Geometry: final body of the model. Coordinates: model frame, mm. Face numbers are marked on the shaded views. Coordinates: 2 decimals unless noted, no trailing zeros. Write each loop counter-clockwise with the first axis right and the second up, starting at its lowest first coordinate (ties: lowest second). Pieces come first, ordered by that corner, then holes. Notation, with made-up numbers: (46, 76) -> (53, 76) arc R28 ccw to (53, 95) -> close; hole circle Ø11 at (31, 0). An arc over 180 degrees is marked (long way). One line per item, written item: value.
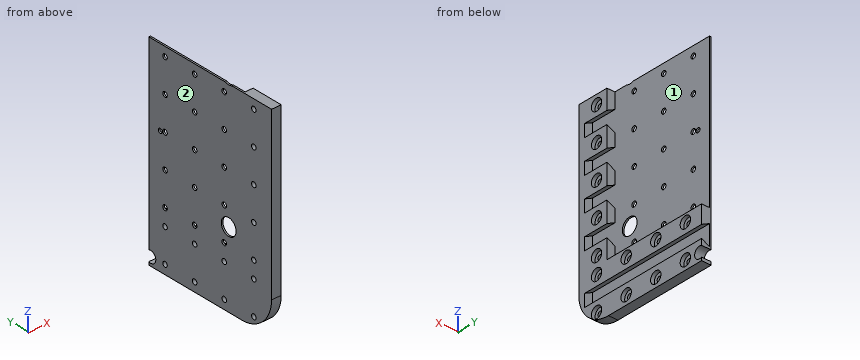
Autodesk Inventor part; units mm, degrees
ref_plane "YZ Plane" through (0, 0, 0) normal (1, 0, 0) x (0, 1, 0)
ref_plane "XZ Plane" through (0, 0, 0) normal (0, 1, 0) x (-1, 0, 0)
ref_plane "XY Plane" through (0, 0, 0) normal (0, 0, 1) x (1, 0, 0)
sketch "Sketch1" plane through (0, 0, 0) normal (0, 1, 0) x (-1, 0, 0)
  line L0 (7.366, 6.1452) -> (7.366, -23.8548)
  line L1 (7.366, -23.8548) -> (0, -23.8548)
  line L2 (6.096, -8.0476) -> (6.096, -9.0212)
  line L3 (0, 0.4868) -> (0, 3.5348)
  line L4 (6.096, 3.5348) -> (6.096, -8.0476)
  line L5 (0, -9.0212) -> (0, -11.8152)
  line L6 (6.096, -12.0692) -> (6.096, -9.0212)
  line L7 (6.096, 3.5348) -> (0, 0.4868)
  line L8 (6.096, -12.0692) -> (0, -9.0212)
  line L9 (0, -23.8548) -> (0, -9.0212)
  line L10 (0, 0.4868) -> (0, 16.3788)
  line L11 (6.096, 13.3308) -> (6.096, 16.3788)
  line L12 (6.096, 13.3308) -> (0, 16.3788)
  line L13 (6.096, 28.9348) -> (6.096, 17.3524)
  line L14 (6.096, 28.9348) -> (0, 25.8868)
  line L15 (6.096, 17.3524) -> (6.096, 16.3788)
  line L16 (6.096, 38.7308) -> (6.096, 41.7788)
  line L17 (6.096, 38.7308) -> (0, 41.7788)
  line L18 (6.096, 54.3348) -> (6.096, 42.7524)
  line L19 (6.096, 54.3348) -> (0, 51.2868)
  line L20 (6.096, 42.7524) -> (6.096, 41.7788)
  line L21 (6.096, 64.1308) -> (6.096, 67.1788)
  line L22 (6.096, 64.1308) -> (0, 67.1788)
  line L23 (6.096, 79.7348) -> (6.096, 68.1524)
  line L24 (6.096, 79.7348) -> (0, 76.6868)
  line L25 (6.096, 68.1524) -> (6.096, 67.1788)
  line L26 (7.366, 6.1452) -> (7.366, 91.622)
  line L27 (7.366, 91.622) -> (0, 91.622)
  line L28 (0, 25.8868) -> (0, 41.7788)
  line L29 (0, 51.2868) -> (0, 67.1788)
  line L30 (0, 76.6868) -> (0, 91.622)
  line L31 (6.096, -4.2672) -> (4.0009, -4.2672) construction
  point P0 (0, 0)
  dimension "d0" = 7.366
  dimension "d8" = 9.508
  dimension "d10" = 3.048
  dimension "d11" = 3.048
  dimension "d12" = 6.096
  dimension "d17" = 25.4
  dimension "d24" = 11.7856
  dimension "d67" = 115.4768
  dimension "d70" = 23.8548
  dimension "d71" = 4.754
extrude "MultipleTeeth" add sketch "Sketch1" along normal blind 19.05
sketch "Sketch2" plane through (0, 0, 0) normal (0, -1, 0) x (1, 0, 0)
  line L0 (0, 0.4868) -> (-6.096, 3.5348) construction
  line L1 (-6.096, 3.5348) -> (-6.096, -12.0692) construction
  line L2 (-6.096, -12.0692) -> (0, -9.0212) construction
  line L3 (0, 16.3788) -> (0, 0.4868)
  line L4 (0, 0.4868) -> (-6.096, 3.5348)
  line L5 (-6.096, -12.0692) -> (0, -9.0212)
  line L6 (-6.096, 3.5348) -> (-6.096, -12.0692)
  line L7 (-6.096, -12.0692) -> (-6.096, 3.5348)
  line L8 (0, -9.0212) -> (-6.096, -12.0692)
  line L9 (-7.366, -23.8548) -> (-7.366, 91.622)
  line L10 (-7.366, -59.508) -> (-7.366, -32.8548)
  line L11 (-7.366, -23.8548) -> (0, -23.8548)
  line L12 (-7.366, 91.622) -> (0, 91.622)
  line L13 (-7.366, -55.8503) -> (-7.366, -40.458) construction
  line L14 (0, -43.0234) -> (0, -59.508) construction
  line L15 (-6.096, -62.0648) -> (0, -62.0648) construction
  line L16 (0, -32.8548) -> (0, -37.6258)
  line L17 (0, -49.9828) -> (0, -62.0648)
  line L18 (0, -62.0648) -> (0, -59.508)
  line L19 (0, -32.8548) -> (-7.366, -32.8548) construction
  line L20 (0, -51.9048) -> (-7.366, -51.9048) construction
  line L21 (0, -42.3798) -> (-7.366, -42.3798) construction
  line L22 (-6.096, -12.0692) -> (-6.096, -62.0648) construction
  line L23 (0, -37.6258) -> (-6.096, -34.5778)
  line L24 (-6.096, -50.1818) -> (-6.096, -34.5778)
  line L25 (0, -47.1338) -> (-6.096, -50.1818)
  line L26 (0, -9.0212) -> (0, -23.8548)
  line L27 (0, -23.8548) -> (0, -32.8548)
  line L28 (-7.366, -32.8548) -> (-7.366, -23.8548)
  line L29 (0, -49.9828) -> (0, -47.1338)
  line L30 (0, -62.0648) -> (-7.366, -62.0648)
  line L31 (-7.366, -62.0648) -> (-7.366, -59.508)
  point P0 (0, 0)
  dimension "d25" = 115.4768
  dimension "d33" = 9
  dimension "d34" = 19.05
  dimension "d36" = 9.525
  dimension "d38" = 10.16
extrude "LongTooth" add sketch "Sketch2" against normal blind 100.2792
sketch "Sketch3" plane through (0, 19.05, 0) normal (0, 1, 0) x (1, 0, 0)
  line L0 (-6.096, -3.5348) -> (-6.096, 12.0692) construction
  line L1 (0, 23.8548) -> (-7.366, 23.8548)
  line L2 (-7.366, -91.622) -> (0, -91.622)
  line L3 (-7.366, 23.8548) -> (-6.096, 23.8548)
  line L4 (-6.096, 23.8548) -> (-6.096, -91.622)
  line L5 (-6.096, -91.622) -> (-7.366, -91.622)
  line L6 (-7.366, -91.622) -> (-7.366, 23.8548)
  point P0 (0, 0)
extrude "ThinPlate" add sketch "Sketch3" along normal up to surface (81.2292 mm away)
sketch "Sketch4" plane through (0, 0, 0) normal (0, -1, 0) x (1, 0, 0)
  line L0 (-6.096, 91.622) -> (0, 91.622)
  line L1 (-7.366, 91.622) -> (-7.366, -62.0648)
  line L2 (0, 91.622) -> (-7.366, 91.622)
  line L3 (-7.366, 91.622) -> (-7.366, -62.0648)
  line L4 (-7.366, -62.0648) -> (0, -62.0648)
  line L5 (0, -62.0648) -> (0, 91.622)
  point P0 (0, 0)
extrude "Extrusion4" add sketch "Sketch4" along normal blind 5.08
ref_plane "Work Plane1" through (-15.892, 0, 8.4328) normal (0, 0, 1) x (0, 1, 0)
sketch "Sketch6" plane through (0, 19.05, 16.3788) normal (1, 0, 0) x (0, 0, -1)
  circle A0 centre (71.4586, -8.89) radius 1.9304
  line L0 (78.4436, -24.13) -> (78.4436, 81.2292)
  line L1 (78.4436, -24.13) -> (-75.2432, -24.13)
  circle A1 centre (58.7586, -8.89) radius 1.9304
  circle A2 centre (46.0586, -8.89) radius 1.9304
  circle A3 centre (71.4586, 3.81) radius 1.9304
  circle A4 centre (58.7586, 3.81) radius 1.9304
  circle A5 centre (46.0586, 3.81) radius 1.9304
  circle A6 centre (71.4586, 16.51) radius 1.9304
  circle A7 centre (58.7586, 16.51) radius 1.9304
  circle A8 centre (46.0586, 16.51) radius 1.9304
  circle A9 centre (71.4586, 29.21) radius 1.9304
  circle A10 centre (58.7586, 29.21) radius 1.9304
  circle A11 centre (46.0586, 29.21) radius 1.9304
  circle A12 centre (71.4586, 41.91) radius 1.9304
  circle A13 centre (58.7586, 41.91) radius 1.9304
  circle A14 centre (46.0586, 41.91) radius 1.9304
  circle A15 centre (71.4586, 54.61) radius 1.9304
  circle A16 centre (58.7586, 54.61) radius 1.9304
  circle A17 centre (46.0586, 54.61) radius 1.9304
  circle A18 centre (71.4586, 67.31) radius 1.9304
  circle A19 centre (58.7586, 67.31) radius 1.9304
  circle A20 centre (46.0586, 67.31) radius 1.9304
  circle A21 centre (33.3586, -8.89) radius 1.9304
  circle A22 centre (33.3586, 3.81) radius 1.9304
  circle A23 centre (33.3586, 16.51) radius 1.9304
  circle A24 centre (33.3586, 29.21) radius 1.9304
  circle A25 centre (33.3586, 41.91) radius 1.9304
  circle A26 centre (33.3586, 54.61) radius 1.9304
  circle A27 centre (33.3586, 67.31) radius 1.9304
  circle A28 centre (20.6586, -8.89) radius 1.9304
  circle A29 centre (20.6586, 3.81) radius 1.9304
  circle A30 centre (20.6586, 16.51) radius 1.9304
  circle A31 centre (20.6586, 29.21) radius 1.9304
  circle A32 centre (20.6586, 41.91) radius 1.9304
  circle A33 centre (20.6586, 54.61) radius 1.9304
  circle A34 centre (20.6586, 67.31) radius 1.9304
  circle A35 centre (7.9586, -8.89) radius 1.9304
  circle A36 centre (7.9586, 3.81) radius 1.9304
  circle A37 centre (7.9586, 16.51) radius 1.9304
  circle A38 centre (7.9586, 29.21) radius 1.9304
  circle A39 centre (7.9586, 41.91) radius 1.9304
  circle A40 centre (7.9586, 54.61) radius 1.9304
  circle A41 centre (7.9586, 67.31) radius 1.9304
  circle A42 centre (-4.7414, -8.89) radius 1.9304
  circle A43 centre (-4.7414, 3.81) radius 1.9304
  circle A44 centre (-4.7414, 16.51) radius 1.9304
  circle A45 centre (-4.7414, 29.21) radius 1.9304
  circle A46 centre (-4.7414, 41.91) radius 1.9304
  circle A47 centre (-4.7414, 54.61) radius 1.9304
  circle A48 centre (-4.7414, 67.31) radius 1.9304
  circle A49 centre (-17.4414, -8.89) radius 1.9304
  circle A50 centre (-17.4414, 3.81) radius 1.9304
  circle A51 centre (-17.4414, 16.51) radius 1.9304
  circle A52 centre (-17.4414, 29.21) radius 1.9304
  circle A53 centre (-17.4414, 41.91) radius 1.9304
  circle A54 centre (-17.4414, 54.61) radius 1.9304
  circle A55 centre (-17.4414, 67.31) radius 1.9304
  circle A56 centre (-30.1414, -8.89) radius 1.9304
  circle A57 centre (-30.1414, 3.81) radius 1.9304
  circle A58 centre (-30.1414, 16.51) radius 1.9304
  circle A59 centre (-30.1414, 29.21) radius 1.9304
  circle A60 centre (-30.1414, 41.91) radius 1.9304
  circle A61 centre (-30.1414, 54.61) radius 1.9304
  circle A62 centre (-30.1414, 67.31) radius 1.9304
  circle A63 centre (-42.8414, -8.89) radius 1.9304
  circle A64 centre (-42.8414, 3.81) radius 1.9304
  circle A65 centre (-42.8414, 16.51) radius 1.9304
  circle A66 centre (-42.8414, 29.21) radius 1.9304
  circle A67 centre (-42.8414, 41.91) radius 1.9304
  circle A68 centre (-42.8414, 54.61) radius 1.9304
  circle A69 centre (-42.8414, 67.31) radius 1.9304
  circle A70 centre (-55.5414, -8.89) radius 1.9304
  circle A71 centre (-55.5414, 3.81) radius 1.9304
  circle A72 centre (-55.5414, 16.51) radius 1.9304
  circle A73 centre (-55.5414, 29.21) radius 1.9304
  circle A74 centre (-55.5414, 41.91) radius 1.9304
  circle A75 centre (-55.5414, 54.61) radius 1.9304
  circle A76 centre (-55.5414, 67.31) radius 1.9304
  circle A77 centre (-68.2414, -8.89) radius 1.9304
  circle A78 centre (-68.2414, 3.81) radius 1.9304
  circle A79 centre (-68.2414, 16.51) radius 1.9304
  circle A80 centre (-68.2414, 29.21) radius 1.9304
  circle A81 centre (-68.2414, 41.91) radius 1.9304
  circle A82 centre (-68.2414, 54.61) radius 1.9304
  circle A83 centre (-68.2414, 67.31) radius 1.9304
  point P0 (16.3788, -19.05)
  dimension "d56" = 3.8608
  dimension "d57" = 6.985
  dimension "d58" = 15.24
  dimension "d61" = 12.7
  dimension "d64" = 12.7
extrude "Extrusion5" cut sketch "Sketch6" against normal through all contours A0 | A2 | A6 | A8 | A12 | A14 | A18 | A20 | A21 | A23 | A25 | A27 | A35 | A37 | A39 | A41 | A49 | A51 | A53 | A55 | A63 | A65 | A67 | A69 | A77 | A79 | A81 | A83
sketch "Sketch7" plane through (0, 19.05, 16.3788) normal (1, 0, 0) x (0, 0, -1)
  circle A0 centre (-68.2414, -8.89) radius 1.9304
  circle A1 centre (-68.2414, -8.89) radius 4.445
  circle A2 centre (-42.8414, -8.89) radius 1.9304
  circle A3 centre (-42.8414, -8.89) radius 4.445
  circle A4 centre (-17.4414, -8.89) radius 1.9304
  circle A5 centre (-17.4414, -8.89) radius 4.445
  circle A6 centre (7.9586, -8.89) radius 1.9304
  circle A7 centre (7.9586, -8.89) radius 4.445
  circle A8 centre (33.3586, -8.89) radius 1.9304
  circle A9 centre (33.3586, -8.89) radius 4.445
  circle A10 centre (46.0586, -8.89) radius 1.9304
  circle A11 centre (46.0586, -8.89) radius 4.445
  circle A12 centre (71.4586, -8.89) radius 1.9304
  circle A13 centre (71.4586, -8.89) radius 4.445
  circle A14 centre (46.0586, 16.51) radius 1.9304
  circle A15 centre (46.0586, 16.51) radius 4.445
  circle A16 centre (71.4586, 16.51) radius 1.9304
  circle A17 centre (71.4586, 16.51) radius 4.445
  circle A18 centre (46.0586, 41.91) radius 1.9304
  circle A19 centre (46.0586, 41.91) radius 4.445
  circle A20 centre (71.4586, 41.91) radius 1.9304
  circle A21 centre (71.4586, 41.91) radius 4.445
  circle A22 centre (46.0586, 67.31) radius 1.9304
  circle A23 centre (46.0586, 67.31) radius 4.445
  circle A24 centre (71.4586, 67.31) radius 4.445
  point P0 (16.3788, -19.05)
  dimension "d74" = 8.89
  dimension "d75" = 8.89
  dimension "d76" = 8.89
  dimension "d77" = 8.89
  dimension "d78" = 8.89
  dimension "d79" = 8.89
  dimension "d80" = 8.89
  dimension "d81" = 8.89
  dimension "d82" = 8.89
  dimension "d83" = 8.89
  dimension "d84" = 8.89
  dimension "d85" = 8.89
  dimension "d86" = 8.89
extrude "Extrusion6" cut sketch "Sketch7" against normal blind 2.8194 contours A0 | A1 | A2 | A3 | A4 | A5 | A6 | A7 | A8 | A9 | A10 | A11 | A12 | A13 | A14 | A15 | A16 | A17 | A18 | A19 | A20 | A21 | A22 | A23 | A24
sketch "Sketch9" plane through (0, 19.05, 16.3788) normal (1, 0, 0) x (0, 0, -1)
  line L0 (78.4436, 81.2292) -> (78.4436, -24.13)
  line L1 (78.4436, -24.13) -> (78.4436, 1.27)
  line L2 (78.4436, -24.13) -> (53.0436, -24.13)
  line L3 (78.4436, -24.13) -> (-75.2432, -24.13)
  arc A0 (53.0436, -24.13) -> (78.4436, 1.27) centre (53.0436, 1.27) ccw
  point P0 (16.3788, -19.05)
  dimension "d91" = 25.4
  dimension "d92" = 25.4
extrude "Extrusion8" cut sketch "Sketch9" against normal through all
sketch "Sketch10" plane through (0, 19.05, 16.3788) normal (1, 0, 0) x (0, 0, -1)
  circle A0 centre (72.0936, 79.5602) radius 1.7 construction
  circle A1 centre (72.0936, 79.5602) radius 4.318
  point P0 (16.3788, -19.05)
  dimension "d95" = 8.636
extrude "Extrusion9" cut sketch "Sketch10" against normal through all
sketch "Sketch11" plane through (-6.096, 19.05, 91.622) normal (1, 0, 0) x (0, 0, -1)
  circle A0 centre (58.7868, 71.4102) radius 1.7 construction
  circle A1 centre (58.7868, 71.4102) radius 1.7
  point P0 (91.622, -19.05)
extrude "Extrusion10" cut sketch "Sketch11" against normal through all
sketch "Sketch12" plane through (-6.096, 19.05, 91.622) normal (1, 0, 0) x (0, 0, -1)
  circle A0 centre (96.2679, 12.7) radius 6.8834 construction
  circle A1 centre (96.2679, 12.7) radius 6.35
  circle A2 centre (-5.7385, 12.6271) radius 5 construction
  circle A3 centre (-5.7385, 12.6271) radius 6.35
  point P0 (91.622, -19.05)
  dimension "d100" = 12.7
  dimension "d101" = 12.7
extrude "Extrusion11" cut sketch "Sketch12" against normal blind 25.4
equation "\"d11\" = d10"
equation "\"d71\" = 0.5 * d8"
equation "\"d36\" = 0.5 * d34"
properties part number "Lift mount receiver left front for metal drive train"
(1) Pull-direction query (Z, two-part tool) for the marked faces 1 and 2; classes: released by +Z, released by -Z, zero draft, split by the parting line, or undercut.
Responses:
face 1: undercut
face 2: zero draft
(2) Line query: line 1 (Z direction, x = -3, y = 87); line 2 (Y direction, x = -0.5, z = -30.5); line 3 (X direction, y = 43.5, z = 56). Output: solid intervals per line, ascending. Write a range as [from, to].
Responses:
line 1: z = [-62.06, -56.9], [-53.26, -48.63], [-36.13, -31.5], [-27.86, -23.85]
line 2: y = [-5.08, 5.79], [14.53, 31.19], [39.93, 56.59], [65.33, 81.99], [90.73, 100.28]
line 3: x = [-7.37, -6.1]
(3) Section A-A (y = 42.5). Return the cut outline in (x, z).
Responses:
outline: (-7.37, -62.06) -> (0, -62.06) -> (0, -47.13) -> (-6.1, -50.18) -> (-6.1, -34.58) -> (0, -37.63) -> (0, -23.85) -> (-6.1, -23.85) -> (-6.1, 91.62) -> (-7.37, 91.62) -> close
(4) Section B-B (z = 44). Return the cut outline in (x, y), then the cut area to 3 significant figures.
Responses:
outline: (-7.37, -5.08) -> (0, -5.08) -> (0, 0) -> (-6.1, 0) -> (-6.1, 100.28) -> (-7.37, 100.28) -> close
area: 165 mm2
(5) First-contact query: pin 1 (5 mm diameter, centred on y = 86.36, z = 33.82, fed in from -X); pin 2 (4 mm diameter, centred on y = 31.5, z = 33.5, fed in from +X); pin 3 (3 mm diameter, centred on x = -1, y = 47.5, fed in from +Z); pin 4 (5.5 mm diameter, centred on y = 10.16, z = 84.62, fed in from +X). Flat tips, straight axial feed; report the tip coordinate or a pass-through.
Responses:
pin 1: stops at x = -7.37
pin 2: stops at x = -6.1
pin 3: stops at z = -23.85
pin 4: stops at x = -2.82
(6) Section C-C (y = 86.36). State how many separate pieces and enclosed holes the cut face has, then the cut area to 3 significant figures.
Responses:
separate pieces: 8
enclosed holes: 0
area: 242 mm2
